from build123d import *

# Parameters (mm, degrees)
EXTRUDE_1_DEPTH = 15


with BuildPart() as part:
    # 草图2 → 凸台-拉伸1 (new body)
    with BuildSketch(Plane.XY.offset(15)):
        with BuildLine():
            Line((0, -22.5), (240, -22.5))
            ThreePointArc((240, -22.5), (262.5, 0), (240, 22.5))
            Line((240, 22.5), (0, 22.5))
            ThreePointArc((0, 22.5), (-22.5, 0), (0, -22.5))
        make_face()
    extrude(amount=-EXTRUDE_1_DEPTH)

    # 草图3 → 切除-旋转1 (revolve, cut)
    with BuildSketch(Plane.XZ, mode=Mode.PRIVATE) as cut_revolve_1_sk:
        Polygon((250.65, 15), (240, 15), (240, 0), (250.65, 0), (250.65, 1), (249.65, 1), (249.65, 6.2), (245.15, 6.2), (245.15, 8.8), (249.65, 8.8), (249.65, 14), (250.65, 14), align=None)
    revolve(cut_revolve_1_sk.sketch.rotate(Axis((240, 0, 15), (0, 0, -1)), 180), axis=Axis((240, 0, 15), (0, 0, -1)), mode=Mode.SUBTRACT)

    # 草图4 → 切除-旋转2 (revolve, cut)
    with BuildSketch(Plane.XZ, mode=Mode.PRIVATE) as cut_revolve_2_sk:
        Polygon((10.65, 15), (0, 15), (0, 0), (10.65, 0), (10.65, 1), (9.65, 1), (9.65, 6.2), (5.15, 6.2), (5.15, 8.8), (9.65, 8.8), (9.65, 14), (10.65, 14), align=None)
    revolve(cut_revolve_2_sk.sketch.rotate(Axis((0, 0, 15), (0, 0, -1)), 180), axis=Axis((0, 0, 15), (0, 0, -1)), mode=Mode.SUBTRACT)


solid = part.part
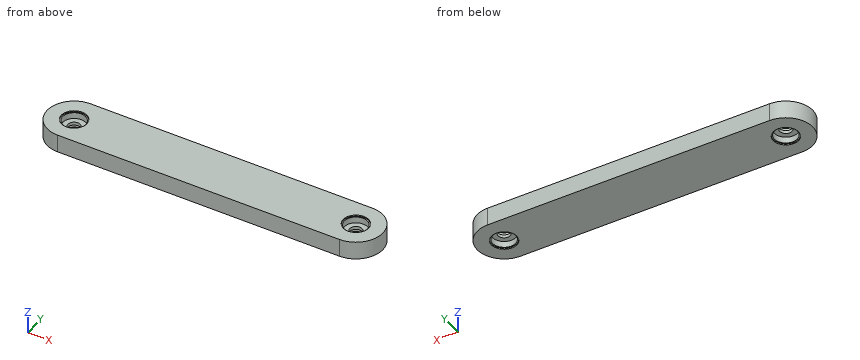
The model under review builds one solid part; all positions refer to its coordinate system, in mm. Coordinates: 2 decimals unless noted, no trailing zeros. Loops run counter-clockwise (first coordinate to the right, second up) from the corner with the lowest first, then second, coordinate; pieces in that order, holes last. Notation, with made-up numbers: (7, 83.5) -> (49, 83.5) arc R9 ccw to (49, 99.5) -> close; hole circle Ø11 at (-9.75, -14). An arc over 180 degrees is marked (long way). Use a Markdown table: item, result. Add a question column.
1. To check wall thickness, follow line 1 (Y direction, x = 0, z = 10.1); line 2 (Y direction, x = 0, z = 0.6); line 3 (X direction, y = -4, z = 2.5). State the ranges of each line that lie inside material, in increasing order.
2. Add section B-B on y = 19. Write out the cut boundary in (x, z).
3. Add section A-A on y = 0. Give the number of separate pieces and of enclosed holes in the cut face, plus the area to 3 significant figures.
4. Clearance check with flat-ended pins moving along their axes: pin 1 Ø17 at (x, y) = (0, 0) entering from -Z; pin 2 Ø15.5 at (x, y) = (238.5, -1.5) entering from -Z; pin 3 Ø17 at (x, y) = (-1.5, -1) entering from +Z; pin 4 Ø9.5 at (x, y) = (240, 0) entering from +Z. State where each tip first meets the part, or that it passes through.
Returned:
| question | item | result |
|---|---|---|
| 1 | line 1 | y = -22.5 to -9.65, 9.65 to 22.5 |
| 1 | line 2 | y = -22.5 to -10.65, 10.65 to 22.5 |
| 1 | line 3 | x = -22.14 to -8.78, 8.78 to 231.22, 248.78 to 262.14 |
| 2 | outline | (-12.05, 0) -> (252.05, 0) -> (252.05, 15) -> (-12.05, 15) -> close |
| 3 | separate pieces | 3 |
| 3 | enclosed holes | 0 |
| 3 | area | 3,730 mm² |
| 4 | pin 1 | stops at z = 6.2 |
| 4 | pin 2 | stops at z = 1 |
| 4 | pin 3 | stops at z = 14 |
| 4 | pin 4 | passes through |
